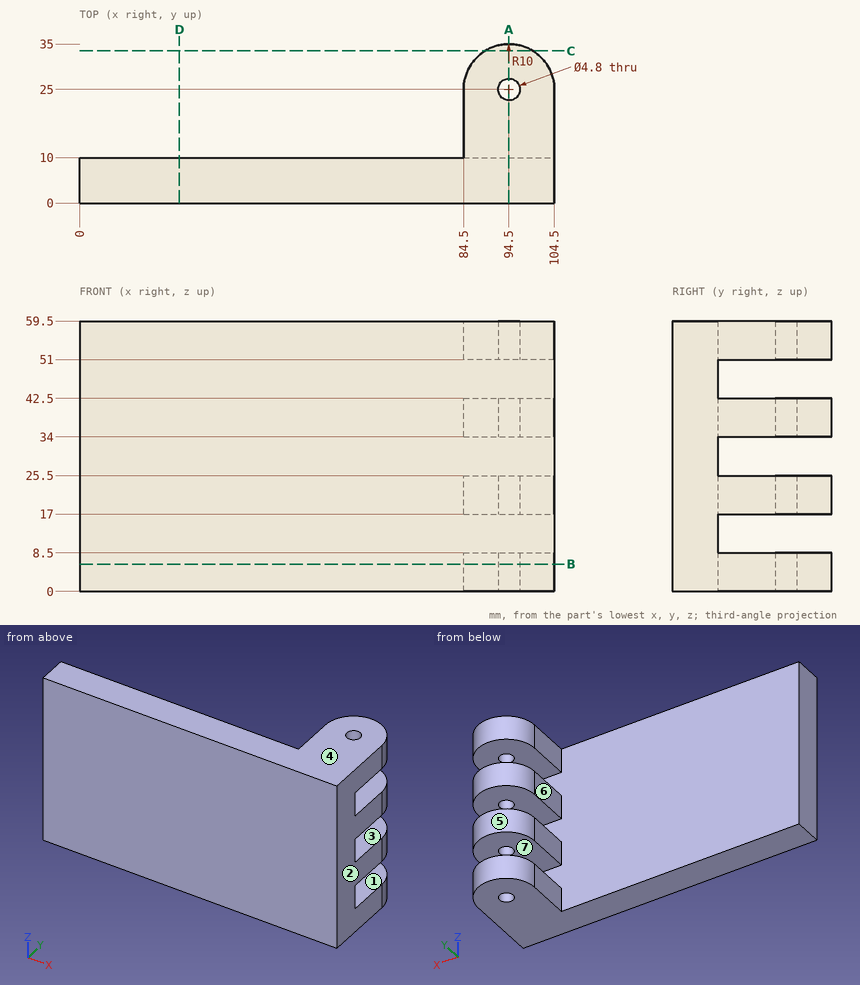
Verification items for this drawing (mm, ordinates from the low corner). A direction names the side the tool comes from. Coordinates: 2 decimals unless noted, no trailing zeros. Write each loop counter-clockwise with the first axis right and the second up, starting at its lowest first coordinate (ties: lowest second). Pieces come first, ordered by that corner, then holes. Notation, with made-up numbers: M -13.75,15.25 L 23.25,15.25 A35 ccw 23.25,51.25 Z; hole C -12.75,-15 d9. An arc over 180 degrees is marked long. Answer as a JSON object with one key per item and string values. Group by question number.
(1) Cross-section at A-A, the plane x = 94.5. State how many separate pieces and enclosed holes the cut face has, and give its area (3 significant figures).
(2) Material ranges on line 1 (Z direction, x = 98, y = 21.5); line 2 (Y direction, x = 94.5, z = 3.5); line 3 (Y direction, x = 76, z = 10.5), recorded low to high.
(3) Release check for a two-part mould opening along Z. For the marked faces 1, 2, 3 and 4 record: +Z half, -Z half, draft (parallel to the pull), parting line (faces both ways), or undercut.
(4) Tool access check on the marked faces 5, 6 and 7. Record the directions out of +Z, -Z, +X, -X, +Y, -Y that give a thin tool (end or side, any length) a straight path to the whole face; none if there is none.
(5) Gauge pin test, flat ends, axial feed: pin 1 (7 mm diameter, centred on y = 20, z = 38, fed in from -X); pin 2 (12 mm diameter, centred on x = 63.5, z = 24.5, fed in from +Y). Record the tip position at first contact, or that the pin passes through.
(6) Cross-section at C-C, the plane y = 33.5. Record the cut outline in (x, z).
(7) Cross-section at B-B, the plane z = 6. Record the cut outline in (x, y).
(8) Cross-section at D-D, the plane x = 22. Record the cut outline in (y, z).
Reply:
{
 "1": {"separate pieces": "5", "enclosed holes": "0", "area": "1,280 mm²"},
 "2": {"line 1": "0 to 8.5, 17 to 25.5, 34 to 42.5, 51 to 59.5", "line 2": "0 to 22.6, 27.4 to 35", "line 3": "0 to 10"},
 "3": {"face 1": "undercut", "face 2": "draft", "face 3": "undercut", "face 4": "+Z half"},
 "4": {"face 5": "+Z, -Z, +Y", "face 6": "+Z, -Z, -X, +Y", "face 7": "+X, -X, +Y"},
 "5": {"pin 1": "x = 84.5", "pin 2": "y = 10"},
 "6": {"outline": "M 89.23,0 L 99.77,0 L 99.77,8.5 L 89.23,8.5 Z; M 89.23,17 L 99.77,17 L 99.77,25.5 L 89.23,25.5 Z; M 89.23,34 L 99.77,34 L 99.77,42.5 L 89.23,42.5 Z; M 89.23,51 L 99.77,51 L 99.77,59.5 L 89.23,59.5 Z"},
 "7": {"outline": "M 0,0 L 104.5,0 L 104.5,25 A10 ccw 84.5,25 L 84.5,10 L 0,10 Z; hole C 94.5,25 d4.8"},
 "8": {"outline": "M 0,0 L 10,0 L 10,59.5 L 0,59.5 Z"}
}
